Part model, mm, in its own coordinate system. A direction names the side the tool comes from. Give positions to 0.01 mm unless a question says otherwise; leave off trailing zeros. Order: outer loops, then holes, each group sorted by start corner. A loop starts at its lowest first (then second) coordinate and runs counter-clockwise, first axis right, second up. Notation, with made-up numbers: M 13,-10 L 28,-10 A11 ccw 28,-2 Z; hole C 61.5,33.5 d7. An arc over 180 degrees is marked long. Return JSON: item names as keys, results as strings.
from build123d import *

# Parameters (mm, degrees)
SKETCH2_W               = 101.6
SKETCH2_H               = 6.35
BOSS_EXTRUDE1_DEPTH     = 152.4
CUT_EXTRUDE1_START      = -6.35
SKETCH3_R               = 6.985
CUT_EXTRUDE1_DEPTH      = 157.289355631
CUT_EXTRUDE2_START      = -6.35
SKETCH4_W               = 101.6
SKETCH4_H               = 38.1
CUT_EXTRUDE2_DEPTH      = 157.815347501
FILLET4_R               = 2.54
SKETCH5_W               = 15.7
SKETCH5_H               = 6
BOSS_EXTRUDE2_DEPTH     = 15.24
SKETCH6_R               = 0.8
CUT_EXTRUDE4_DEPTH      = 176.555716512
FILLET7_R               = 0.762
FILLET8_R               = 0.762
TAP_DRILL_FOR_M2_TAP3_D = 1.6


with BuildPart() as part:
    # Sketch2 → Boss-Extrude1 (new body)
    with BuildSketch(Plane.XY):
        with BuildLine():
            Line((-50.8, -3.175), (-5.335878714, -24.224686475))
            ThreePointArc((-5.335878714, -24.224686475), (0, -25.4), (5.335878714, -24.224686475))
            Line((5.335878714, -24.224686475), (50.8, -3.175))
            Line((50.8, -3.175), (-50.8, -3.175))
        make_face()
        Rectangle(SKETCH2_W, SKETCH2_H)
    extrude(amount=BOSS_EXTRUDE1_DEPTH)

    # Sketch3 → Cut-Extrude1 (cut, through all)
    with BuildSketch(Plane.XY.offset(152.4).offset(CUT_EXTRUDE1_START)):
        with Locations((0, -12.7)):
            Circle(SKETCH3_R)
    extrude(amount=-CUT_EXTRUDE1_DEPTH, mode=Mode.SUBTRACT)

    # Sketch4 → Cut-Extrude2 (cut, through all)
    with BuildSketch(Plane(origin=(0, 3.175, 0), x_dir=(1, 0, 0), z_dir=(0, 1, 0)).offset(CUT_EXTRUDE2_START)):
        with Locations((0, -76.2)):
            Rectangle(SKETCH4_W, SKETCH4_H)
    extrude(amount=-CUT_EXTRUDE2_DEPTH, mode=Mode.SUBTRACT)

    # Fillet4
    fillet4_edges = [part.edges().sort_by_distance(p)[0] for p in [
        (-50.8, 3.175, 76.2),
        (50.8, 3.175, 76.2),
    ]]
    fillet(fillet4_edges, radius=FILLET4_R)

    # Sketch5 → Boss-Extrude2 (add)
    with BuildSketch(Plane(origin=(0, 3.175, 0), x_dir=(1, 0, 0), z_dir=(0, 1, 0))):
        with Locations((40.41, -98.6)):
            Rectangle(SKETCH5_W, SKETCH5_H)
        with Locations((40.41, -69.6)):
            Rectangle(SKETCH5_W, SKETCH5_H)
    extrude(amount=BOSS_EXTRUDE2_DEPTH)

    # Sketch6 → Cut-Extrude4 (cut, through all)
    with BuildSketch(Plane.ZY.offset(-32.56)):
        with Locations((97.995000084, 15.875)):
            Circle(SKETCH6_R)
        with Locations((70.204999916, 15.875)):
            Circle(SKETCH6_R)
    extrude(amount=-CUT_EXTRUDE4_DEPTH, mode=Mode.SUBTRACT)

    # Fillet7
    fillet7_edges = [part.edges().sort_by_distance(p)[0] for p in [
        (40.41, 18.415, 95.6),
        (40.41, 18.415, 101.6),
    ]]
    fillet(fillet7_edges, radius=FILLET7_R)

    # Fillet8
    fillet8_edges = [part.edges().sort_by_distance(p)[0] for p in [
        (40.41, 18.415, 66.6),
        (40.41, 18.415, 72.6),
    ]]
    fillet(fillet8_edges, radius=FILLET8_R)

    # Tap Drill for M2 Tap3 (through all)
    with Locations(Plane.ZY.offset(-32.56)):
        with Locations((97.995000084, 15.875), (70.204999916, 15.875)):
            Hole(TAP_DRILL_FOR_M2_TAP3_D / 2)


solid = part.part
Q1. Band-saw the part on C-C (z = 137). Give the cut face in (x, y) (3 decimals), then the cut area to 3 significant figures.
Established:
{"outline": "M -50.8,-3.175 L -5.336,-24.225 A12.7 ccw 5.336,-24.225 L 50.8,-3.175 L 50.8,0.635 A2.54 ccw 48.26,3.175 L -48.26,3.175 A2.54 ccw -50.8,0.635 Z; hole C 0,-12.7 d13.97", "area": "1,680 mm²"}
Q2. Probe line 1 along Y through (x, z) = (0, 134) (3 decimals); line 2 along Z through (x, y) = (5.5, -21); line 3 along Y through (x, z) = (-12, 85) (3 decimals). List the from-to ranges inside material, lowest first.
Established:
{"line 1": "y = -25.4 to -19.685, -5.715 to 3.175", "line 2": "z = 0 to 57.15, 95.25 to 152.4", "line 3": "y = -3.175 to 3.175"}
Q3. Band-saw the part on B-B (y = 8). Give the cut face in (x, z).
Established:
{"outline": "M 32.56,66.6 L 48.26,66.6 L 48.26,72.6 L 32.56,72.6 Z; M 32.56,95.6 L 48.26,95.6 L 48.26,101.6 L 32.56,101.6 Z"}
Q4. Pin check, flat tips, straight feed: pin 1 (6 mm diameter, centred on x = -15, z = 122, fed in from -Y); pin 2 (5 mm diameter, centred on x = 29.5, z = 29.5, fed in from +Y) (3 decimals); pin 3 (8 mm diameter, centred on y = -13.5, z = 46.5, fed in from +X); pin 4 (1.3 mm diameter, centred on y = 15.875, z = 70.205, fed in from +X). Stop position of each tip, or through.
Established:
{"pin 1": "stops at y = -21.14", "pin 2": "stops at y = 3.175", "pin 3": "stops at x = 37.14", "pin 4": "passes through"}
Q5. 3-axis set-ups, long thin cutter, end or side, ignore diameter. For faces 4 (the flat face through (40, 10, 72.6)), 5 (the flat face through (32.56, 11, 99)), 6 (the flat face through (-1, -3.175, 76)), 7 (the flat face through (0, -13, 146.05)), 8 (the flat face through (48.26, 11, 70)): which of +Z, -Z, +X, -X, +Y, -Y reach the whole face in a straight line?
Established:
{"face 4": "+X, -X, +Y", "face 5": "+Z, -Z, -X, +Y", "face 6": "+X, -X, -Y", "face 7": "-Z", "face 8": "+Z, -Z, +X, +Y"}
Q6. Two-plate mould, pull along Z, no slides. Class faces 1 (the flat face through (40, 10, 95.6)), 2 (the flat face through (32.56, 11, 70)), 3 (the flat face through (40, 10, 66.6)): +Z half, -Z half, draft (parallel to the pull), parting line (faces both ways), or undercut.
Established:
{"face 1": "undercut", "face 2": "draft", "face 3": "-Z half"}
Q7. Band-saw the part on D-D (y = -12.7). Give the cut face in (x, z) (3 decimals).
Established:
{"outline": "M -30.227,0 L -6.985,0 L -6.985,57.15 L -30.227,57.15 Z; M -30.227,95.25 L -6.985,95.25 L -6.985,146.05 L 6.985,146.05 L 6.985,95.25 L 30.227,95.25 L 30.227,152.4 L -30.227,152.4 Z; M 6.985,0 L 30.227,0 L 30.227,57.15 L 6.985,57.15 Z"}
Q8. Band-saw the part on A-A (x = 0). Give the cut face in (y, z) (3 decimals).
Established:
{"outline": "M -25.4,0 L -19.685,0 L -19.685,57.15 L -25.4,57.15 Z; M -25.4,95.25 L -19.685,95.25 L -19.685,146.05 L -5.715,146.05 L -5.715,95.25 L -3.175,95.25 L -3.175,57.15 L -5.715,57.15 L -5.715,0 L 3.175,0 L 3.175,152.4 L -25.4,152.4 Z"}
